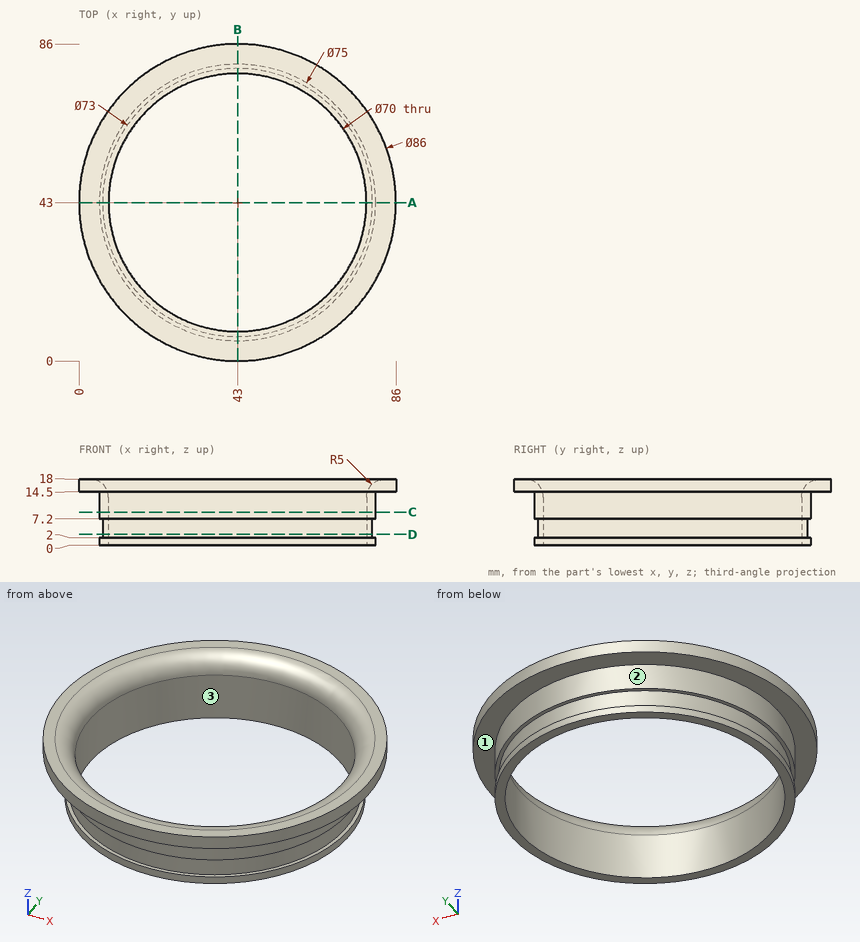
The drawing under review shows one solid part. Ordinate dimensions are in mm from its lowest x, y, z. Round coordinates to 2 decimals unless told otherwise and drop trailing zeros. Write each loop counter-clockwise with the first axis right and the second up, starting at its lowest first coordinate (ties: lowest second). Pieces come first, ordered by that corner, then holes. Notation, with made-up numbers: M -14,29 L 36,29 A14 cw 36,54 Z; hole C -21.75,48 d3. An arc over 180 degrees is marked long. One line per item, written item: value. Start each with the question number.
(1) We need section C-C (z = 9). Give the boundary of the cut face in (x, y).
(2) Wall thickness on line 1 (Y direction, x = 43, z = 5); line 2 (X direction, y = 41, z = 3.75); line 3 (Y direction, x = 43, z = 8.5): over which ranges is each line inside the solid? List them lowest first.
(3) We need section D-D (z = 3). Give the boundary of the cut face in (x, y).
(4) The part is to be moulded in two halves that separate along Y. For the marked faces 1, 2 and 3, say which applies: released by +Y, released by -Y, zero draft, split by the parting line, or undercut.
(5) We need section A-A (y = 43). Give the boundary of the cut face in (x, z), and give its area (3 significant figures).
(6) Insertion check: pin 1 (10 mm diameter, centred on x = 20, z = 14.5, fed in from +Y); pin 2 (6 mm diameter, centred on x = 16, z = 3, fed in from -Y); pin 3 (4 mm diameter, centred on y = 42, z = 12, fed in from +X). Each pin has a flat end and moves straight along its axis. Give the tip position at first contact, or say it passes through.
Result:
1. outline: C 43,43 d75; hole C 43,43 d70
2. line 1: 6.5 to 8, 78 to 79.5
2. line 2: 6.55 to 8.06, 77.94 to 79.45
2. line 3: 5.5 to 8, 78 to 80.5
3. outline: C 43,43 d73; hole C 43,43 d70
4. face 1: zero draft
4. face 2: split by the parting line
4. face 3: undercut
5. outline: M 0,14.5 L 5.5,14.5 L 5.5,7.2 L 6.5,7.2 L 6.5,2 L 5.5,2 L 5.5,0 L 8,0 L 8,13 A5 ccw 3,18 L 0,18 Z; M 78,0 L 80.5,0 L 80.5,2 L 79.5,2 L 79.5,7.2 L 80.5,7.2 L 80.5,14.5 L 86,14.5 L 86,18 L 83,18 A5 ccw 78,13 Z
5. area: 107 mm²
6. pin 1: y = 82.05
6. pin 2: y = 14.33
6. pin 3: x = 80.5
